Autodesk Inventor part; units mm, degrees
ref_plane "YZ Plane" through (0, 0, 0) normal (1, 0, 0) x (0, 1, 0)
ref_plane "XZ Plane" through (0, 0, 0) normal (0, 1, 0) x (-1, 0, 0)
ref_plane "XY Plane" through (0, 0, 0) normal (0, 0, 1) x (1, 0, 0)
sketch "Sketch1" plane through (0, 0, 0) normal (0, 0, 1) x (1, 0, 0)
  line L0 (-16, -12.5) -> (16, -12.5)
  line L1 (16, -12.5) -> (16, 12.5)
  line L2 (16, 12.5) -> (13, 12.5)
  line L3 (13, 12.5) -> (13, -9.5)
  line L4 (13, -9.5) -> (-13, -9.5)
  line L5 (-13, -9.5) -> (-13, 12.5)
  line L6 (-13, 12.5) -> (-16, 12.5)
  line L7 (-16, 12.5) -> (-16, -12.5)
  point P0 (0, 0)
  dimension "d0" = 32
  dimension "d1" = 25
  dimension "d2" = 3
  dimension "d3" = 90
  dimension "d4" = 22
  dimension "d5" = 26
  dimension "d6" = 22
  dimension "d7" = 3
  dimension "d8" = 25
  dimension "d10" = 12.5
  dimension "d11" = 16
extrude "Extrusion1" add sketch "Sketch1" against normal blind 609.6
chamfer "Chamfer1" distance 25 angle 30 1 edges at (14.5, 12.5, 0) measured on face at (4.3333, -11.5, 0)
chamfer "Chamfer2" distance 25 angle 30 1 edges at (14.5, 12.5, -609.6) measured on face at (4.3333, -11.5, -609.6)
sketch "Sketch3" plane through (16, -12.5, 0) normal (1, 0, 0) x (0, 0, -1)
  line L0 (595.1662, 25) -> (609.6, 0)
  line L1 (14.4338, 25) -> (595.1662, 25)
  line L2 (0, 0) -> (14.4338, 25)
  line L3 (0, 0) -> (609.6, 0)
  line L4 (0, 12.5) -> (609.6, 12.5) construction
  line L5 (68.9831, 0) -> (83.4169, 25) construction
  line L6 (526.1831, 25) -> (540.6169, 0) construction
  circle A0 centre (76.2, 12.5) radius 3.175
  circle A1 centre (533.4, 12.5) radius 3.175
  dimension "d62" = 6.35
  dimension "d63" = 6.35
  dimension "d64" = 76.2
  dimension "d65" = 76.2
hole "Hole4" at (16, 0, -76.2) at (16, 0, -533.4) direction (-1, 0, 0) diameter 6.35 depth 3 tip angle 118
equation "\"d5\" = d0 - 2 * d2"
equation "\"d65\" = d64"
properties part number "Chassis Rear Edge"
The model under review builds one solid part; all positions refer to its coordinate system, in mm. A direction names the side the tool comes from. Round coordinates to 2 decimals unless told otherwise and drop trailing zeros. Loops run counter-clockwise (first coordinate to the right, second up) from the corner with the lowest first, then second, coordinate; pieces in that order, holes last. Notation, with made-up numbers: (21.25, 0.25) - (72.25, 0.25) arc R26 ccw to (72.25, 32.25) - close; hole circle Ø10 at (-34, 81). An arc over 180 degrees is marked (long way). Use a Markdown table: item, result. Add a question column.
Q1. Insertion check: pin 1 Ø10 at (x, y) = (-10, 9.5) entering from +Z; pin 2 Ø10 at (x, z) = (-11.5, -446.5) entering from +Y; pin 3 Ø13 at (x, z) = (0, -218) entering from +Y. Each pin has a flat end and moves straight along its axis. Give the tip position at first contact, or say it passes through.
Q2. Add section A-A (z = -309). State the section outline as (x, y) points.
Q3. The part is to be moulded in two halves that separate along X. For faces 3 (the face through (-1.26, -10.13, -1.37)), 4 (the face through (16, 0, -301)), 5 (the face through (-13, 1, -301)), say which applies: pulls with the +X half, pulls with the -X half, needs draft (parallel to the pull), parting line crosses it, or undercut.
Q4. For probe 1 along X at (y, z) = (3.75, -192); probe 2 along Y at (x, z) = (14, -76); probe 3 along Z at (x, y) = (13.9, 0) (3 decimals), list the stretches that pass through material, from the lowest coordinate up.
Q5. Machinability: for faces 1 (the face through (0, -12.5, -301)), 2 (the face through (0, -9.5, -301)), which of the approach directions +Z, -Z, +X, -X, +Y, -Y give a long, thin tool a straight path to every point of the face, cutting with its end or side? Answer none if there is none.
Worked answers:
| question | item | result |
|---|---|---|
| 1 | pin 1 | z = -10.39 |
| 1 | pin 2 | y = 12.5 |
| 1 | pin 3 | y = -9.5 |
| 2 | outline | (-16, -12.5) - (16, -12.5) - (16, 12.5) - (13, 12.5) - (13, -9.5) - (-13, -9.5) - (-13, 12.5) - (-16, 12.5) - close |
| 3 | face 3 | needs draft |
| 3 | face 4 | pulls with the +X half |
| 3 | face 5 | undercut |
| 4 | probe 1 | -16 to -13, 13 to 16 |
| 4 | probe 2 | -12.5 to -3.17, 3.17 to 12.5 |
| 4 | probe 3 | -602.384 to -536.575, -530.225 to -79.375, -73.025 to -7.216 |
| 5 | face 1 | +Z, -Z, +X, -X, -Y |
| 5 | face 2 | +Z, -Z, +Y |
